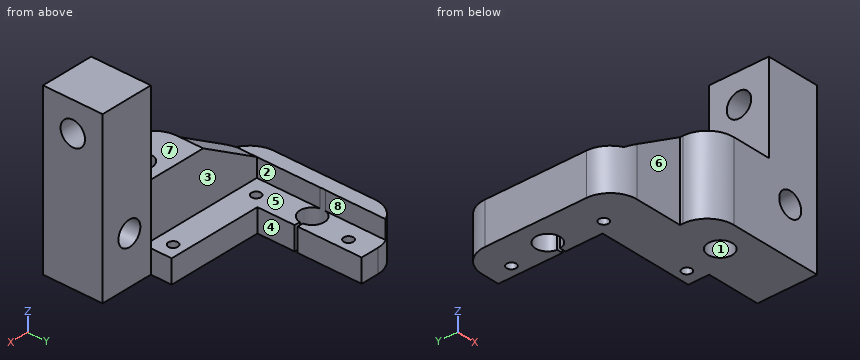
from build123d import *

# Parameters (mm, degrees)
PAD_DEPTH       = 56
SKETCH001_W     = 42
SKETCH001_H     = 48.2
POCKET_DEPTH    = 44.2
SKETCH002_R     = 1.6
SKETCH002_R_2   = 4.1
POCKET001_DEPTH = 56.001
SKETCH003_R     = 4.1
POCKET002_DEPTH = 20.001
SKETCH004_W     = 5
SKETCH004_H     = 42
POCKET003_DEPTH = 62.001
POCKET004_DEPTH = 62.001
SKETCH006_R     = 4.1
POCKET005_DEPTH = 65.001
FILLET_R        = 9


with BuildPart() as part:
    # Sketch → Pad (new body)
    with BuildSketch(Plane(origin=(0, 0, 0), x_dir=(1, 0, 0), z_dir=(0, 0, -1))):
        Polygon((-50, 40), (-10, 40), (-10, 20), (-28, 20), (-28, -22), (-75, -22), (-75, 30), (-50, 30), align=None)
    extrude(amount=PAD_DEPTH)

    # Sketch001 → Pocket (cut)
    with BuildSketch(Plane(origin=(0, 22, 0), x_dir=(1, 0, 0), z_dir=(0, 1, 0))):
        with Locations((-49, 24.1)):
            Rectangle(SKETCH001_W, SKETCH001_H)
    extrude(amount=-POCKET_DEPTH, mode=Mode.SUBTRACT)

    # Sketch002 → Pocket001 (cut, through all)
    with BuildSketch(Plane(origin=(0, 0, -56), x_dir=(1, 0, 0), z_dir=(0, 0, -1))):
        with Locations((-33, 17)):
            Circle(SKETCH002_R)
        with Locations((-64, 17)):
            Circle(SKETCH002_R)
        with Locations((-64, -14)):
            Circle(SKETCH002_R)
        with Locations((-35, 30)):
            Circle(SKETCH002_R_2)
        with BuildLine():
            Line((-60, 13), (-28, 13))
            Line((-28, 13), (-28, -22))
            Line((-60, -22), (-28, -22))
            Line((-60, -22), (-60, -0.5))
            Line((-61.930602, -0.5), (-60, -0.5))
            ThreePointArc((-61.930602, 0.5), (-70.1, 0), (-61.930602, -0.5))
            Line((-61.930602, 0.5), (-60, 0.5))
            Line((-60, 13), (-60, 0.5))
        make_face()
    extrude(amount=-POCKET001_DEPTH, mode=Mode.SUBTRACT)

    # Sketch003 → Pocket002 (cut, through all)
    with BuildSketch(Plane(origin=(0, -20, 0), x_dir=(1, 0, 0), z_dir=(0, 1, 0))):
        with Locations((-20, 40)):
            Circle(SKETCH003_R)
    extrude(amount=-POCKET002_DEPTH, mode=Mode.SUBTRACT)

    # Sketch004 → Pocket003 (cut, through all)
    with BuildSketch(Plane(origin=(0, 22, 0), x_dir=(1, 0, 0), z_dir=(0, 1, 0))):
        with Locations((-72.5, 21)):
            Rectangle(SKETCH004_W, SKETCH004_H)
    extrude(amount=-POCKET003_DEPTH, mode=Mode.SUBTRACT)

    # Sketch005 → Pocket004 (cut, through all)
    with BuildSketch(Plane(origin=(0, -40, 0), x_dir=(-1, 0, 0), z_dir=(0, -1, 0))):
        Polygon((28, 0), (28, 30), (50, 30), (70, 42), (70, 0), align=None)
    extrude(amount=-POCKET004_DEPTH, mode=Mode.SUBTRACT)

    # Sketch006 → Pocket005 (cut, through all)
    with BuildSketch(Plane(origin=(-10, 0, 0), x_dir=(0, -1, 0), z_dir=(1, 0, 0))):
        with Locations((30, 10)):
            Circle(SKETCH006_R)
    extrude(amount=-POCKET005_DEPTH, mode=Mode.SUBTRACT)

    # Fillet
    fillet_edges = [part.edges().sort_by_distance(p)[0] for p in [
        (-75, 22, -49),
        (-75, -30, -49),
        (-50, -40, -43),
    ]]
    fillet(fillet_edges, radius=FILLET_R)


solid = part.part
Can you work these out from the model? Positions are in its coordinate system, mm. Face numbers are marked on the shaded views. A direction names the side the tool comes from. Coordinates: 2 decimals unless noted, no trailing zeros. Write each loop counter-clockwise with the first axis right and the second up, starting at its lowest first coordinate (ties: lowest second). Pieces come first, ordered by that corner, then holes. Notation, with made-up numbers: (1, 22) -> (52, 22) arc R7 ccw to (52, 28) -> close; hole circle Ø9 at (5, 29.25). An arc over 180 degrees is marked (long way). Write each question's results on one line, items separated by ' | '. Start each with the question number.
Q1. Imagine slicing it at B-B (z = -10). Write out the boundary of the cut face in (x, y), then the cut area to 3 significant figures.
Q2. Imagine slicing it at D-D (y = 14). Write out the boundary of the cut face in (x, z).
Q3. On a 3-axis mill with a long thin cutter (end or side, diameter ignored), from which of +Z, -Z, +X, -X, +Y, -Y can I reach the whole of each face in a straight line? I mean the marked faces 4, 5, 6, 7 and 8. Say none if no direction works.
Q4. I'm going to push flat-ended pins straight in: pin 1 (2.5 mm diameter, centred on y = -5, z = -53, fed in from +X); pin 2 (8 mm diameter, centred on x = -41, y = -6, fed in from -Z); pin 3 (9 mm diameter, centred on x = -19, z = -14.5, fed in from +Y); pin 4 (7.5 mm diameter, centred on y = -16.5, z = -50.5, fed in from +X). Where does each tip first touch, or does it pass through?
Q5. Imagine slicing it at C-C (x = -25). Write out the boundary of the cut face in (y, z), then the cut area to 3 significant figures.
Q6. Imagine slicing it at A-A (y = -28). Write out the boundary of the cut face in (x, z).
Q7. If I drill on probe 1 along X at (y, z) = (-17, -50.75); probe 2 along Z at (x, y) = (-20, -30); probe 3 along Y at (x, z) = (-64, -54), over which ranges is the centre line in solid material (lowest first)?
Q8. We'd pull the mould along Y, two halves only. Please class the marked faces 1, 2 and 3: +Y half, -Y half, draft (parallel to the pull), parting line (faces both ways), or undercut.
Taken from the geometry:
1) outline: (-28, -40) -> (-10, -40) -> (-10, -34.1) -> (-28, -34.1) -> close; (-28, -25.9) -> (-10, -25.9) -> (-10, -20) -> (-28, -20) -> close | area: 212 mm^2
2) outline: (-74.94, -56) -> (-65.6, -56) -> (-65.6, -48.2) -> (-70, -48.2) -> (-70, -42) -> (-74.94, -42) -> close; (-62.4, -56) -> (-60, -56) -> (-60, -48.2) -> (-62.4, -48.2) -> close
3) face 4: +Z, -Z, +X, +Y | face 5: +Z, +Y | face 6: +Z, -Z, -X, -Y | face 7: +Z, -X, +Y, -Y | face 8: +Z, +X, +Y
4) pin 1: stops at x = -60 | pin 2: passes through | pin 3: stops at y = -20 | pin 4: stops at x = -10
5) outline: (-40, -56) -> (-20, -56) -> (-20, 0) -> (-40, 0) -> close; hole circle Ø8.2 at (-30, -10) | area: 1,070 mm^2
6) outline: (-71.66, -56) -> (-38.58, -56) -> (-38.58, -30) -> (-50, -30) -> (-70, -42) -> (-71.66, -42) -> close; (-31.42, -56) -> (-10, -56) -> (-10, -13.58) -> (-28, -13.58) -> (-28, -30) -> (-31.42, -30) -> close; (-28, -6.42) -> (-10, -6.42) -> (-10, 0) -> (-28, 0) -> close; hole circle Ø8.2 at (-20, -40)
7) probe 1: x = -75 to -65.6, -62.4 to -34.6, -31.4 to -28 | probe 2: z = -56 to -44.1, -35.9 to -14.1, -5.9 to 0 | probe 3: y = -30 to -18.6, -15.4 to -3.58, 3.58 to 12.4, 15.6 to 22
8) face 1: undercut | face 2: draft | face 3: +Y half
